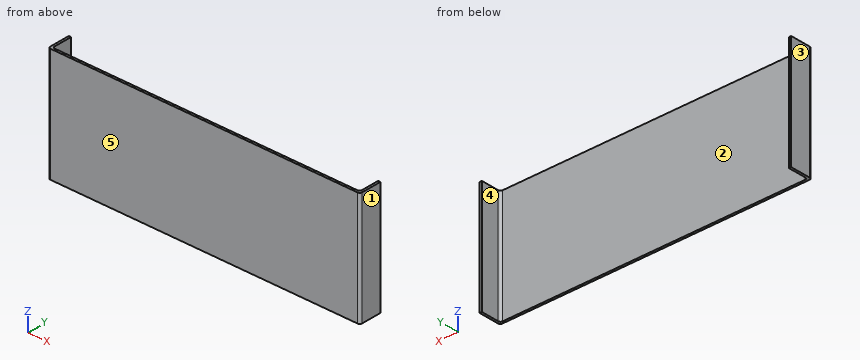
```python
from build123d import *

# Parameters (mm, degrees)
SKETCH1_W           = 275
SKETCH1_H           = 100
BOSS_EXTRUDE1_DEPTH = 20
SHELL2_T            = -2
FILLET1_R           = 2


with BuildPart() as part:
    # Sketch1 → Boss-Extrude1 (new body)
    with BuildSketch(Plane(origin=(0, 0, 0), x_dir=(1, 0, 0), z_dir=(0, 1, 0))):
        with Locations((-137.5, 50)):
            Rectangle(SKETCH1_W, SKETCH1_H)
    extrude(amount=BOSS_EXTRUDE1_DEPTH)

    # Shell2
    shell2_openings = [part.faces().sort_by_distance(p)[0] for p in [
        (-137.5, 20, -50),
        (-137.5, 10, 0),
        (-137.5, 10, -100),
    ]]
    offset(amount=SHELL2_T, openings=shell2_openings, kind=Kind.INTERSECTION)

    # Fillet1
    fillet1_edges = [part.edges().sort_by_distance(p)[0] for p in [
        (-2, 2, -50),
        (-273, 2, -50),
        (-275, 0, -50),
        (0, 0, -50),
    ]]
    fillet(fillet1_edges, radius=FILLET1_R)


solid = part.part
```
The listing builds one solid part. Answer for the finished solid, in the listing's coordinates (mm). Face numbers are marked on the shaded views. A direction names the side the tool comes from. Coordinates: 2 decimals unless noted, no trailing zeros. Loops run counter-clockwise (first coordinate to the right, second up) from the corner with the lowest first, then second, coordinate; pieces in that order, holes last. Notation, with made-up numbers: (-17.75, 79.5) - (-6.75, 79.5) arc R20 cw to (-6.75, 115.5) - close; hole circle Ø8 at (-32.5, -32). An arc over 180 degrees is marked (long way). Use a Markdown table: item, result. Add a question column.
1) The mould has two halves that part along X. Classify the marked faces 3, 4 and 5: released by +X, released by -X, zero draft, split by the parting line, or undercut.
2) Find the intervals of material crossed by line 1 (X direction, y = 17.5, z = -58); line 2 (Y direction, x = -165.5, z = -58.5); line 3 (X direction, y = 1.5, z = -12), in increasing order.
3) For the marked faces 1 and 2, determine the directions among +Z, -Z, +X, -X, +Y, -Y from which every point of the face is accessible in a straight line to the end or side of a thin tool.
4) The part is cut by section A-A, the plane y = 8. Give the vertices of the cut face in (x, z), and give its area (3 significant figures).
5) The part is cut by section C-C, the plane x = -242.5. Give the vertices of the cut face in (y, z), and give its area (3 significant figures).
6) The part is cut by section B-B, the plane z = -82. Give the vertices of the cut face in (x, y).
Here are the results:
| question | item | result |
|---|---|---|
| 1 | face 3 | released by -X |
| 1 | face 4 | undercut |
| 1 | face 5 | zero draft |
| 2 | line 1 | x = -275 to -273, -2 to 0 |
| 2 | line 2 | y = 0 to 2 |
| 2 | line 3 | x = -274.94 to -0.06 |
| 3 | face 1 | +Z, -Z, +X, +Y, -Y |
| 3 | face 2 | +Z, -Z, +Y |
| 4 | outline | (-275, -100) - (-273, -100) - (-273, 0) - (-275, 0) - close; (-2, -100) - (0, -100) - (0, 0) - (-2, 0) - close |
| 4 | area | 400 mm^2 |
| 5 | outline | (0, -100) - (2, -100) - (2, 0) - (0, 0) - close |
| 5 | area | 200 mm^2 |
| 6 | outline | (-275, 2) arc R2 ccw to (-273, 0) - (-2, 0) arc R2 ccw to (0, 2) - (0, 20) - (-2, 20) - (-2, 4) arc R2 cw to (-4, 2) - (-271, 2) arc R2 cw to (-273, 4) - (-273, 20) - (-275, 20) - close |
